Geometry check sheet. Reference: the model listing, model coordinates, mm. A direction names the side the tool comes from. Give positions to 0.01 mm unless a question says otherwise; leave off trailing zeros. Loops run counter-clockwise (first coordinate to the right, second up) from the corner with the lowest first, then second, coordinate; pieces in that order, holes last.
```python
from build123d import *

# Parameters (mm, degrees)
SZKIC1_W                    = 28
SZKIC1_H                    = 33
DODANIE_WYCI_GNI_CIE1_DEPTH = 1.5
SZKIC2_W                    = 28
SZKIC2_H                    = 33
SZKIC2_W_2                  = 20.4
SZKIC2_H_2                  = 29.4
DODANIE_WYCI_GNI_CIE2_DEPTH = 19
SZKIC7_W                    = 20.4
SZKIC7_H                    = 29.4
SZKIC7_W_2                  = 15.6
SZKIC7_H_2                  = 26.6
DODANIE_WYCI_GNI_CIE4_DEPTH = 8.5
SZKIC3_W                    = 12
SZKIC3_H                    = 10.5
WYTNIJ_WYCI_GNI_CIE1_DEPTH  = 3.8
SZKIC4_W                    = 19
SZKIC4_H                    = 8
WYTNIJ_WYCI_GNI_CIE2_DEPTH  = 1.8
SZKIC5_W                    = 11
SZKIC5_H                    = 8
WYTNIJ_WYCI_GNI_CIE3_DEPTH  = 3.8
WYTNIJ_WYCI_GNI_CIE4_START  = -10
WYTNIJ_WYCI_GNI_CIE4_DEPTH  = 10
WYTNIJ_WYCI_GNI_CIE8_START  = -1.5
WYTNIJ_WYCI_GNI_CIE8_DEPTH  = 8.5
ZAOKR_GLENIE1_R             = 2
SZKIC10_W                   = 5.4
SZKIC10_H                   = 7.2
WYTNIJ_WYCI_GNI_CIE9_DEPTH  = 0.4
SZKIC11_W                   = 5.4
SZKIC11_H                   = 2.5
WYTNIJ_WYCI_GNI_CIE10_DEPTH = 1
SZKIC12_W                   = 6
SZKIC12_H                   = 7.2
WYTNIJ_WYCI_GNI_CIE11_DEPTH = 0.4
SZKIC13_W                   = 6
SZKIC13_H                   = 2.5
WYTNIJ_WYCI_GNI_CIE12_DEPTH = 1
SFAZOWANIE1_SIZE            = 1
SFAZOWANIE2_SIZE            = 3
SFAZOWANIE3_SIZE            = 2.5
SFAZOWANIE3_SIZE_2          = 2.979383981


# Some blends are built 0.0001 mm under size
with BuildPart() as part:
    # Szkic1 → Dodanie-wyciągnięcie1 (new body)
    with BuildSketch(Plane(origin=(0, 0, 0), x_dir=(1, 0, 0), z_dir=(0, 1, 0))):
        Rectangle(SZKIC1_W, SZKIC1_H)
    extrude(amount=DODANIE_WYCI_GNI_CIE1_DEPTH)

    # Szkic2 → Dodanie-wyciągnięcie2 (add)
    with BuildSketch(Plane(origin=(0, 1.5, 0), x_dir=(1, 0, 0), z_dir=(0, 1, 0))):
        Rectangle(SZKIC2_W, SZKIC2_H)
        Rectangle(SZKIC2_W_2, SZKIC2_H_2, mode=Mode.SUBTRACT)
    extrude(amount=DODANIE_WYCI_GNI_CIE2_DEPTH)

    # Szkic7 → Dodanie-wyciągnięcie4 (add)
    with BuildSketch(Plane(origin=(0, 1.5, 0), x_dir=(1, 0, 0), z_dir=(0, 1, 0))):
        Rectangle(SZKIC7_W, SZKIC7_H)
        Rectangle(SZKIC7_W_2, SZKIC7_H_2, mode=Mode.SUBTRACT)
    extrude(amount=DODANIE_WYCI_GNI_CIE4_DEPTH)

    # Szkic3 → Wytnij-wyciągnięcie1 (cut)
    with BuildSketch(Plane(origin=(14, 0, 0), x_dir=(0, 0, -1), z_dir=(1, 0, 0))):
        with Locations((7.4, 15.25)):
            Rectangle(SZKIC3_W, SZKIC3_H)
    extrude(amount=-WYTNIJ_WYCI_GNI_CIE1_DEPTH, mode=Mode.SUBTRACT)

    # Szkic4 → Wytnij-wyciągnięcie2 (cut)
    with BuildSketch(Plane.XY.offset(16.5)):
        with Locations((0, 16.5)):
            Rectangle(SZKIC4_W, SZKIC4_H)
    extrude(amount=-WYTNIJ_WYCI_GNI_CIE2_DEPTH, mode=Mode.SUBTRACT)

    # Szkic5 → Wytnij-wyciągnięcie3 (cut)
    with BuildSketch(Plane.ZY.offset(14)):
        with Locations((-7.6, 16.5)):
            Rectangle(SZKIC5_W, SZKIC5_H)
    extrude(amount=-WYTNIJ_WYCI_GNI_CIE3_DEPTH, mode=Mode.SUBTRACT)

    # Szkic8 → Wytnij-wyciągnięcie4 (cut)
    with BuildSketch(Plane.XZ.offset(WYTNIJ_WYCI_GNI_CIE4_START)):
        with BuildLine():
            Line((9.5, 4.35), (4.5, 4.35))
            ThreePointArc((4.5, 4.35), (2.85, 6), (4.5, 7.65))
            Line((4.5, 7.65), (9.5, 7.65))
            ThreePointArc((9.5, 7.65), (11.15, 6), (9.5, 4.35))
        make_face()
        with BuildLine():
            Line((-9.5, 4.35), (-4.5, 4.35))
            ThreePointArc((-4.5, 4.35), (-2.85, 6), (-4.5, 7.65))
            Line((-4.5, 7.65), (-9.5, 7.65))
            ThreePointArc((-9.5, 7.65), (-11.15, 6), (-9.5, 4.35))
        make_face()
    extrude(amount=WYTNIJ_WYCI_GNI_CIE4_DEPTH, mode=Mode.SUBTRACT)

    # Szkic9 → Wytnij-wyciągnięcie8 (cut)
    with BuildSketch(Plane.XZ.offset(WYTNIJ_WYCI_GNI_CIE8_START)):
        with BuildLine():
            Line((-9.5, 2.4), (-5.001731613, 2.4))
            Line((-5.001731613, 2.4), (-5.001731613, 9.6))
            Line((-5.001731613, 9.6), (-9.5, 9.6))
            ThreePointArc((-9.5, 9.6), (-13.1, 6), (-9.5, 2.4))
        make_face()
        with BuildLine():
            Line((5.001731613, 9.6), (9.5, 9.6))
            ThreePointArc((9.5, 9.6), (13.1, 6), (9.5, 2.4))
            Line((9.5, 2.4), (5.001731613, 2.4))
            Line((5.001731613, 2.4), (5.001731613, 9.6))
        make_face()
    extrude(amount=-WYTNIJ_WYCI_GNI_CIE8_DEPTH, mode=Mode.SUBTRACT)

    # Zaokrąglenie1
    zaokr_glenie1_edges = [part.edges().sort_by_distance(p)[0] for p in [
        (12.1, 10, -13.4),
        (12.1, 10, -1.4),
    ]]
    fillet(zaokr_glenie1_edges, radius=ZAOKR_GLENIE1_R)

    # Szkic10 → Wytnij-wyciągnięcie9 (cut)
    with BuildSketch(Plane(origin=(14, 0, 0), x_dir=(0, 0, -1), z_dir=(1, 0, 0))):
        with Locations((-6, 16.9)):
            Rectangle(SZKIC10_W, SZKIC10_H)
    wytnij_wyci_gni_cie9 = extrude(amount=-WYTNIJ_WYCI_GNI_CIE9_DEPTH, mode=Mode.SUBTRACT)

    # Szkic11 → Wytnij-wyciągnięcie10 (cut)
    with BuildSketch(Plane(origin=(13.6, 0, 0), x_dir=(0, 0, -1), z_dir=(1, 0, 0))):
        with Locations((-6, 14.55)):
            Rectangle(SZKIC11_W, SZKIC11_H)
    wytnij_wyci_gni_cie10 = extrude(amount=-WYTNIJ_WYCI_GNI_CIE10_DEPTH, mode=Mode.SUBTRACT)

    # Szkic12 → Wytnij-wyciągnięcie11 (cut)
    with BuildSketch(Plane(origin=(0, 0, -16.5), x_dir=(-1, 0, 0), z_dir=(0, 0, -1))):
        with Locations((0, 16.9)):
            Rectangle(SZKIC12_W, SZKIC12_H)
    extrude(amount=-WYTNIJ_WYCI_GNI_CIE11_DEPTH, mode=Mode.SUBTRACT)

    # Szkic13 → Wytnij-wyciągnięcie12 (cut)
    with BuildSketch(Plane(origin=(0, 0, -16.1), x_dir=(-1, 0, 0), z_dir=(0, 0, -1))):
        with Locations((0, 14.55)):
            Rectangle(SZKIC13_W, SZKIC13_H)
    extrude(amount=-WYTNIJ_WYCI_GNI_CIE12_DEPTH, mode=Mode.SUBTRACT)

    # Lustro1: Wytnij-wyciągnięcie9, Wytnij-wyciągnięcie10 across plane
    add(wytnij_wyci_gni_cie9.mirror(Plane(origin=(0, 0, 0), x_dir=(0, 0, 1), z_dir=(1, 0, 0))), mode=Mode.SUBTRACT)
    add(wytnij_wyci_gni_cie10.mirror(Plane(origin=(0, 0, 0), x_dir=(0, 0, 1), z_dir=(1, 0, 0))), mode=Mode.SUBTRACT)

    # Sfazowanie1
    sfazowanie1_edges = [part.edges().sort_by_distance(p)[0] for p in [
        (12.6, 15.8, 6),
        (0, 15.8, -15.1),
        (-12.6, 15.8, 6),
    ]]
    chamfer(sfazowanie1_edges, length=SFAZOWANIE1_SIZE - 0.0001)  # a hair under: the kernel refuses the full size

    # Sfazowanie2
    sfazowanie2_edges = [part.edges().sort_by_distance(p)[0] for p in [
        (14, 10.25, 16.5),
        (-14, 10.25, 16.5),
    ]]
    chamfer(sfazowanie2_edges, length=SFAZOWANIE2_SIZE)

    # Sfazowanie3
    # the kernel refuses this chamfer: 2.979383981, 2.5 mm, written as the material it adds along each edge
    with BuildSketch(Plane(origin=(9.5, 10, 6), x_dir=(-0.9999950652018581, 0, 0.0031415874858795353), z_dir=(-0.0031415874858795353, 0, -0.9999950652018581))) as sfazowanie3_piece_1_section:
        Polygon((3.6, -SFAZOWANIE3_SIZE), (3.6 - SFAZOWANIE3_SIZE_2, 0), (3.6, 0), align=None)
    sfazowanie3_piece_1 = revolve(axis=Axis((9.5, 10, 6), (0, 1, 0)), revolution_arc=359.64, mode=Mode.PRIVATE)
    sfazowanie3_piece_1 = split(sfazowanie3_piece_1, bisect_by=Plane(origin=(10.2, 9.026977163, 6), z_dir=(1, 0, 0)), keep=Keep.TOP, mode=Mode.PRIVATE)
    add(sfazowanie3_piece_1)
    with BuildSketch(Plane(origin=(-9.5, 10, 6), x_dir=(0.9999950652018581, 0, 0.003141587485879782), z_dir=(0.003141587485879782, 0, -0.9999950652018581))) as sfazowanie3_piece_2_section:
        Polygon((3.6 - SFAZOWANIE3_SIZE_2, 0), (3.6, SFAZOWANIE3_SIZE), (3.6, 0), align=None)
    sfazowanie3_piece_2 = revolve(axis=Axis((-9.5, 10, 6), (0, -1, 0)), revolution_arc=359.64, mode=Mode.PRIVATE)
    sfazowanie3_piece_2 = split(sfazowanie3_piece_2, bisect_by=Plane(origin=(-10.2, 9.026977163, 6.000000001), z_dir=(-1, 0, 0)), keep=Keep.TOP, mode=Mode.PRIVATE)
    add(sfazowanie3_piece_2)


solid = part.part
```
1) Scan lines: line 1 along X through (y, z) = (5.75, -3); line 2 along Z through (x, y) = (-6.5, 6.5); line 3 along Z through (x, y) = (-5.5, 10.5). Record each from-to range of solid material in increasing order.
2) Depth check by flat-ended pin: P1, Ø4, axis at x = 3.5, z = 11.5, coming from the +Y side; P2, Ø8, axis at x = 2.5, z = 4, coming from the -Y side; P3, Ø1.5, axis at x = -13, y = 16, coming from the +Z side; P4, Ø8, axis at x = 3.5, z = 5, coming from the +Y side. Enter the tip coordinate at first touch or a pass-through.
3) Sectioned sample at C-C on y = 2.25. Enter the section's corners in (x, z).
4) Tool access check on faces 1 (the cylindrical face through (-11.15, 0.76, 6.04)), 2 (the cylindrical face through (13.1, 4.7, 6.1)), 3 (the flat face through (13.8, 16, 8.7)), 4 (the flat face through (7.8, 6, 11)). Record the directions out of +Z, -Z, +X, -X, +Y, -Y that give a thin tool (end or side, any length) a straight path to the whole face; none if there is none.
5) Sectioned sample at A-A on x = -5.75. Enter the section's corners in (y, z), plus the area to 3 significant figures.
6) Sectioned sample at B-B on z = 6. Count the separate pieces of the cut face and the enclosed holes in it, plus the area to 3 significant figures.
7) Sectioned sample at D-D on z = 14. Enter the section's corners in (x, y), plus the area to 3 significant figures.
8) Mould release check, pull along X, two halves, no side actions. Record for faces 5 (the flat face through (-14, 8, -1)), 6 (the flat face through (12.6, 14, 6)), 7 (the flat face through (-12, 20.5, 7)), 8 (the flat face through (0, 12.5, 16)): +X half, -X half, draft (parallel to the pull), parting line (faces both ways), or undercut.
Determined:
1. line 1: x = -14 to -7.8, 7.8 to 14
1. line 2: z = -16.5 to -13.3, 13.3 to 16.5
1. line 3: z = -16.5 to -14.7, 14.7 to 16.5
2. P1: stops at y = 10
2. P2: stops at y = 0
2. P3: stops at z = 15.25
2. P4: stops at y = 1.5
3. outline: (-14, -16.5) - (14, -16.5) - (14, 13.5) - (11, 16.5) - (-11, 16.5) - (-14, 13.5) - close; hole (-9.5, 2.4) - (-7.8, 2.4) - (-7.8, -13.3) - (7.8, -13.3) - (7.8, 2.4) - (9.5, 2.4) arc R3.6 ccw to (9.5, 9.6) - (7.8, 9.6) - (7.8, 13.3) - (-7.8, 13.3) - (-7.8, 9.6) - (-9.5, 9.6) arc R3.6 ccw to start
4. face 1: -Y
4. face 2: none
4. face 3: +X
4. face 4: +Y
5. outline: (0, -16.5) - (20.5, -16.5) - (20.5, -14.7) - (10, -14.7) - (10, -13.3) - (1.5, -13.3) - (1.5, 4.35) - (0, 4.35) - close; (0, 7.65) - (1.5, 7.65) - (1.5, 13.3) - (10, 13.3) - (10, 14.7) - (12.5, 14.7) - (12.5, 16.5) - (0, 16.5) - close
5. area: 122 mm2
6. separate pieces: 3
6. enclosed holes: 0
6. area: 110 mm2
7. outline: (-13.5, 0) - (13.5, 0) - (13.5, 20.5) - (10.2, 20.5) - (10.2, 10) - (-10.2, 10) - (-10.2, 20.5) - (-13.5, 20.5) - close
7. area: 339 mm2
8. face 5: -X half
8. face 6: +X half
8. face 7: draft
8. face 8: undercut
